Build history of the part. All positions in model axes, mm. Give positions to 0.01 mm unless a question says otherwise; leave off trailing zeros. Loops run counter-clockwise (first coordinate to the right, second up) from the corner with the lowest first, then second, coordinate; pieces in that order, holes last. Notation, with made-up numbers: M -21,-37.5 L 26,-37.5 A18 cw 26,-9.5 Z; hole C 30,43.5 d11. An arc over 180 degrees is marked long. Put each result on its own line as item: value.
```python
from build123d import *

# Parameters (mm, degrees)
F0_W     = 95.25
F0_H     = 158.75
F0_W_2   = 6.35
F0_H_2   = 133.35
F1_DEPTH = 4.7752
F2_R     = 41.275
F3_DEPTH = 25.4
F4_SIZE  = 3.302


with BuildPart() as f1:
    # F0 (on Top) → F1 (new body)
    with BuildSketch(Plane.XY):
        Polygon((-50.8, -73.025), (50.8, -73.025), (50.8, 60.325), (57.15, 60.325), (57.15, 73.025), (47.625, 73.025), (-47.625, 73.025), (-57.15, 73.025), (-57.15, 60.325), (-50.8, 60.325), align=None)
        with Locations((0, 152.4)):
            Rectangle(F0_W, F0_H)
        with Locations((-53.975, -6.35)):
            Rectangle(F0_W_2, F0_H_2)
        with Locations((53.975, -6.35)):
            Rectangle(F0_W_2, F0_H_2)
    extrude(amount=F1_DEPTH)

    # F2 (on face) → F3 (cut)
    with BuildSketch(Plane.XY.offset(4.7752)):
        Circle(F2_R)
    extrude(amount=-F3_DEPTH, mode=Mode.SUBTRACT)

    # F4
    f4_edges = [f1.edges().sort_by_distance(p)[0] for p in [
        (0, -73.025, 4.7752),
    ]]
    chamfer(f4_edges, length=F4_SIZE)


solid = f1.part
```
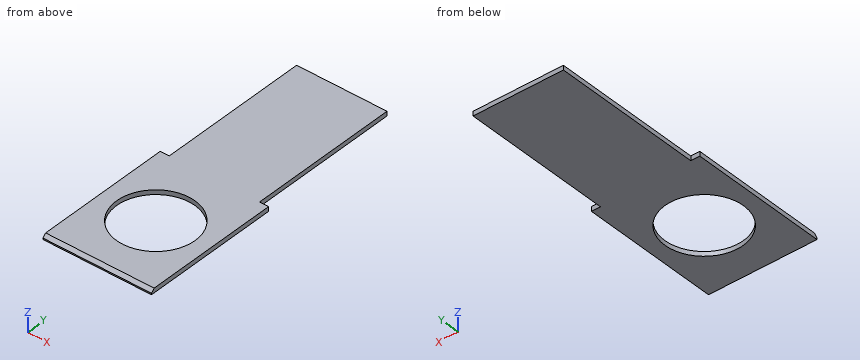
Q1. Probe line 1 (X direction, y = -0.5, z = 3); line 2 (Y direction, x = 0, z = 1.5) (3 decimals); line 3 (X direction, y = 130.5, z = 2.1) (3 decimals). List the from-to ranges inside material, lowest first. Write a range as from..to.
Here are the results:
line 1: -57.15..-41.27, 41.27..57.15
line 2: -72.998..-41.275, 41.275..231.775
line 3: -47.625..47.625
Q2. Slice it at A-A (x = 0). List the corners of the cut face in (y, z) (3 decimals).
Here are the results:
outline: M -73.025,0 L -41.275,0 L -41.275,4.775 L -69.723,4.775 L -73.025,1.473 Z; M 41.275,0 L 231.775,0 L 231.775,4.775 L 41.275,4.775 Z
Q3. Drop flat-ended pins along their axis: pin 1 Ø1.4 at (y, z) = (132, 2) entering from +X (3 decimals); pin 2 Ø2.5 at (y, z) = (151, 3) entering from -X (3 decimals); pin 3 Ø2.5 at (x, z) = (50.5, 1.5) entering from +Y (3 decimals). Give the stop position or say it passes through.
Here are the results:
pin 1: x = 47.625
pin 2: x = -47.625
pin 3: y = 73.025
Q4. Slice it at B-B (y = 0). List the corners of the cut face in (x, z) (3 decimals).
Here are the results:
outline: M -57.15,0 L -41.275,0 L -41.275,4.775 L -57.15,4.775 Z; M 41.275,0 L 57.15,0 L 57.15,4.775 L 41.275,4.775 Z
Q5. Slice it at D-D (x = 31.5). List the corners of the cut face in (y, z) (3 decimals).
Here are the results:
outline: M -73.025,0 L -26.672,0 L -26.672,4.775 L -69.723,4.775 L -73.025,1.473 Z; M 26.672,0 L 231.775,0 L 231.775,4.775 L 26.672,4.775 Z
Q6. Slice it at C-C (z = 3.3). List the corners of the cut face in (x, y) (3 decimals), and give its area (3 significant figures).
Here are the results:
outline: M -57.15,-71.198 L 57.15,-71.198 L 57.15,73.025 L 47.625,73.025 L 47.625,231.775 L -47.625,231.775 L -47.625,73.025 L -57.15,73.025 Z; hole C 0,0 d82.55
area: 26,300 mm²
